from build123d import *

# Parameters (mm, degrees)
BOSS_EXTRUDE1_DEPTH = 3.175
SKETCH2_R           = 4.7625
CUT_EXTRUDE1_DEPTH  = 73.203842884


with BuildPart() as part:
    # Sketch1 → Boss-Extrude1 (new body)
    with BuildSketch(Plane.XY):
        with BuildLine():
            Line((-20.151174843, -15.462540297), (-61.251157558, 38.1))
            Line((-61.251157558, 38.1), (61.251157558, 38.1))
            Line((61.251157558, 38.1), (20.151174843, -15.462540297))
            ThreePointArc((20.151174843, -15.462540297), (0, -25.4), (-20.151174843, -15.462540297))
        make_face()
    extrude(amount=BOSS_EXTRUDE1_DEPTH)

    # Sketch2 → Cut-Extrude1 (cut, through all)
    with BuildSketch(Plane.XY.offset(3.175)):
        Circle(SKETCH2_R)
    extrude(amount=-CUT_EXTRUDE1_DEPTH, mode=Mode.SUBTRACT)


solid = part.part
Source: CAD feature listing. Evaluate the final solid. Frame: model axes, mm. Give positions to 0.01 mm unless a question says otherwise; leave off trailing zeros. Write each loop counter-clockwise with the first axis right and the second up, starting at its lowest first coordinate (ties: lowest second). Pieces come first, ordered by that corner, then holes. Notation, with made-up numbers: (-4, 16.5) -> (32, 16.5) arc R20 ccw to (32, 22.5) -> close; hole circle Ø11 at (63, 70.5). An arc over 180 degrees is marked (long way). Write item = value, one per line.
Q1. Cut plane D-D on x = 26. Return loops of the section in (y, z) (3 decimals).
Here are the results:
outline = (-7.84, 0) -> (38.1, 0) -> (38.1, 3.175) -> (-7.84, 3.175) -> close
Q2. Line query: line 1 (Y direction, x = -1, z = 0.65); line 2 (Y direction, x = 50.5, z = 0.35); line 3 (Y direction, x = -9, z = 2.4). Output: solid intervals per line, ascending. Write a range as from..to.
Here are the results:
line_1 = -25.38..-4.66, 4.66..38.1
line_2 = 24.09..38.1
line_3 = -23.75..38.1
Q3. Cut plane C-C on y = -1.5. Return loops of the section in (x, z) (3 decimals), then the cut area to 3 significant figures.
Here are the results:
outline = (-30.865, 0) -> (-4.52, 0) -> (-4.52, 3.175) -> (-30.865, 3.175) -> close; (4.52, 0) -> (30.865, 0) -> (30.865, 3.175) -> (4.52, 3.175) -> close
area = 167 mm²
Q4. First-contact query: pin 1 (1 mm diameter, centred on x = -12.5, z = 0.5, fed in from -Y); pin 2 (5 mm diameter, centred on x = 26, y = -14, fed in from +Z). Flat tips, straight axial feed; report the tip coordinate or a pass-through.
Here are the results:
pin_1 = -22.39
pin_2 = through
Q5. Cut plane A-A on x = 0. Return loops of the section in (y, z) (1 decimal).
Here are the results:
outline = (-25.4, 0) -> (-4.8, 0) -> (-4.8, 3.2) -> (-25.4, 3.2) -> close; (4.8, 0) -> (38.1, 0) -> (38.1, 3.2) -> (4.8, 3.2) -> close
Q6. Cut plane B-B on z = 1.7. Return loops of the section in (x, y) (1 decimal).
Here are the results:
outline = (-61.3, 38.1) -> (-20.2, -15.5) arc R25.4 ccw to (20.2, -15.5) -> (61.3, 38.1) -> close; hole circle Ø9.5 at (0, 0)
Q7. Mould query, pull axis Y, two halves, no side actions, for faces 1 (the face through (-3.78, -2.9, 1.61)), 2 (the face through (40.989, 11.694, 1.565)), 3 (the face through (-1, 38.1, 2)), 4 (the face through (1, 14, 0)). Classes: +Y half, -Y half, draft (parallel to the pull), parting line (faces both ways), or undercut.
Here are the results:
face_1 = undercut
face_2 = -Y half
face_3 = +Y half
face_4 = draft
